Design review of the part shown in the three views and the two pictorial views. Dimensions are in mm from the part's minimum x, y and z. A direction names the side the tool comes from. Round coordinates to 2 decimals unless told otherwise and drop trailing zeros. Order: outer loops, then holes, each group sorted by start corner. A loop starts at its lowest first (then second) coordinate and runs counter-clockwise, first axis right, second up. Notation, with made-up numbers: M -5,80.5 L 16,80.5 A32 ccw 16,115.5 Z; hole C 8.25,36 d8. An arc over 180 degrees is marked long. Write item = value, one per line. Start each with the question number.
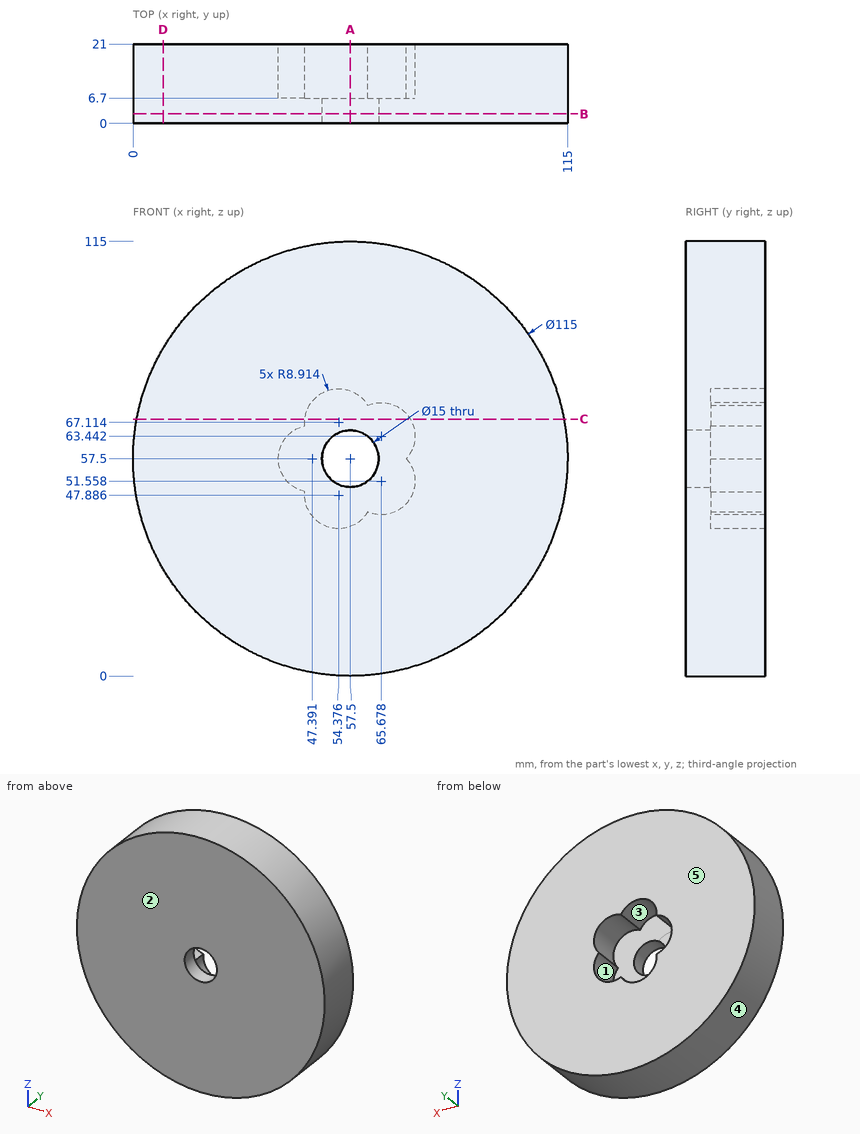
(1) We need section A-A, the plane x = 57.5. Write out the cut boundary in (y, z), then the cut area to 3 significant figures.
(2) Insertion check: pin 1 (12 mm diameter, centred on x = 57.5, z = 57.5, fed in from -Y); pin 2 (6 mm diameter, centred on x = 99.5, y = 15, fed in from -Z); pin 3 (1 mm diameter, centred on x = 18.5, y = 18, fed in from -Z); pin 4 (1 mm diameter, centred on x = 76, y = 6, fed in from +Z). Each pin has a flat end and moves straight along its axis. Give the tip position at first contact, or say it passes through.
(3) For the marked faces 1 and 2, list the 3-axis set-ups (+Z, -Z, +X, -X, +Y, -Y) from which the entire face can be reached by the end or side of a thin tool; tool diameter is ignored.
(4) We need section D-D, the plane x = 8. Write out the cut boundary in (y, z), then the cut area to 3 significant figures.
(5) Draft analysis for pull direction X (two halves, no side actions). For the marked faces 3, 4 and 5, state which applies: released by +X, released by -X, zero draft, split by the parting line, or undercut.
(6) For line 1 along X through (y, z) = (1.75, 57.5); line 2 along X through (y, z) = (11.25, 41) (1 decimal); line 3 along Y through (x, z) = (68, 56.5), list the stretches that pass through material, from the lowest coordinate up.
(7) We need section C-C, the plane z = 68. Write out the cut boundary in (x, y).
(8) We need section B-B, the plane y = 2.5. Write out the cut boundary in (x, z).
Values:
q1.outline = M 0,0 L 21,0 L 21,39.54 L 6.7,39.54 L 6.7,50 L 0,50 Z; M 0,65 L 6.7,65 L 6.7,75.46 L 21,75.46 L 21,115 L 0,115 Z
q1.area = 1,800 mm²
q2.pin_1 = through
q2.pin_2 = 15.25
q2.pin_3 = 14.79
q2.pin_4 = 112.11
q3.face_1 = +Y
q3.face_2 = +Z, -Z, +X, -X, -Y
q4.outline = M 0,28.24 L 21,28.24 L 21,86.76 L 0,86.76 Z
q4.area = 1,230 mm²
q5.face_3 = undercut
q5.face_4 = split by the parting line
q5.face_5 = zero draft
q6.line_1 = 0 to 50, 65 to 115
q6.line_2 = 2.4 to 48.7, 60 to 112.6
q6.line_3 = 0 to 6.7
q7.outline = M 0.97,0 L 114.03,0 L 114.03,21 L 73.34,21 L 73.34,6.7 L 45.51,6.7 L 45.51,21 L 0.97,21 Z
q8.outline = C 57.5,57.5 d115; hole C 57.5,57.5 d15
